Answer from the drawing. Dimensions are ordinates in mm from the lowest x, y and z of the part. Round coordinates to 2 decimals unless told otherwise and drop trailing zeros. Loops run counter-clockwise (first coordinate to the right, second up) from the corner with the lowest first, then second, coordinate; pieces in that order, holes last. Notation, with made-up numbers: M -35.75,65 L 23.25,65 A16 cw 23.25,74 Z; hole C 34,88.5 d8. An arc over 180 degrees is marked long. Answer as a JSON object with one key per item and string values.
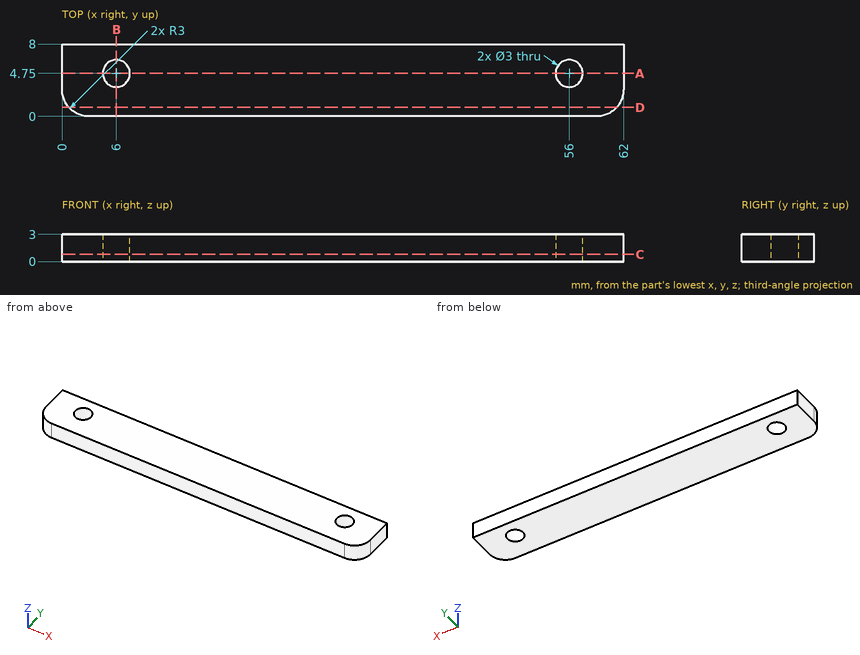
Item 1: The part is cut by section B-B (x = 6). Give the vertices of the cut face in (y, z), then the cut area to 3 significant figures.
Values follow:
{"outline": "M 0,0 L 3.25,0 L 3.25,3 L 0,3 Z; M 6.25,0 L 8,0 L 8,3 L 6.25,3 Z", "area": "15.0 mm^2"}
Item 2: Flat-ended cylindrical pins translate along their axes: P1, Ø1, axis at y = 1, z = 1.5, coming from the -X side; P2, Ø1.8, axis at x = 6, y = 4.75, coming from the -Z side; P3, Ø3.5, axis at x = 56, y = 4.75, coming from the -Z side. Find the tip coordinate at first contact, or state that the pin passes through.
Values follow:
{"P1": "x = 0.4", "P2": "through", "P3": "z = 0"}
Item 3: The part is cut by section D-D (y = 1). Give the vertices of the cut face in (x, z), then the cut area to 3 significant figures.
Values follow:
{"outline": "M 0.76,0 L 61.24,0 L 61.24,3 L 0.76,3 Z", "area": "181 mm^2"}
Item 4: The part is cut by section A-A (y = 4.75). Give the vertices of the cut face in (x, z), then the cut area to 3 significant figures.
Values follow:
{"outline": "M 0,0 L 4.5,0 L 4.5,3 L 0,3 Z; M 7.5,0 L 54.5,0 L 54.5,3 L 7.5,3 Z; M 57.5,0 L 62,0 L 62,3 L 57.5,3 Z", "area": "168 mm^2"}
Item 5: Straight lines are drawn through the part: line 1 (Y direction, x = 56, z = 1); line 2 (X direction, y = 5, z = 0.85); line 3 (X direction, y = 2.75, z = 2.8). For each, find the intervals that lie inside material, in ascending order.
Values follow:
{"line 1": "0 to 3.25, 6.25 to 8", "line 2": "0 to 4.52, 7.48 to 54.52, 57.48 to 62", "line 3": "0.01 to 61.99"}
Item 6: The part is cut by section C-C (z = 0.8). Give the vertices of the cut face in (x, y).
Values follow:
{"outline": "M 0,3 A3 ccw 3,0 L 59,0 A3 ccw 62,3 L 62,8 L 0,8 Z; hole C 6,4.75 d3; hole C 56,4.75 d3"}
